```python
from build123d import *

# Parameters (mm, degrees)
SKETCH1_R           = 6.4
BOSS_EXTRUDE1_DEPTH = 77.83
SKETCH2_OUTSIDE_W   = 30.782
SKETCH2_OUTSIDE_H   = 30.782
SKETCH2_OUTSIDE_R   = 3.9
CUT_EXTRUDE1_DEPTH  = 70
CUT_EXTRUDE2_DEPTH  = 5.64
FILLET1_R           = 0.5


with BuildPart() as part:
    # Sketch1 → Boss-Extrude1 (new body)
    with BuildSketch(Plane(origin=(0, 0, 0), x_dir=(1, 0, 0), z_dir=(0, 1, 0))):
        Circle(SKETCH1_R)
    extrude(amount=BOSS_EXTRUDE1_DEPTH)

    # Sketch2 outside → Cut-Extrude1 (cut)
    with BuildSketch(Plane(origin=(0, 77.83, 0), x_dir=(1, 0, 0), z_dir=(0, 1, 0))):
        Rectangle(SKETCH2_OUTSIDE_W, SKETCH2_OUTSIDE_H)
        Circle(SKETCH2_OUTSIDE_R, mode=Mode.SUBTRACT)
    extrude(amount=-CUT_EXTRUDE1_DEPTH, mode=Mode.SUBTRACT)

    # Sketch8 → Cut-Extrude2 (cut)
    with BuildSketch(Plane.XZ):
        Polygon((3.464101615, 0), (1.732050808, 3), (-1.732050808, 3), (-3.464101615, 0), (-1.732050808, -3), (1.732050808, -3), align=None)
    extrude(amount=-CUT_EXTRUDE2_DEPTH, mode=Mode.SUBTRACT)

    # Fillet1
    fillet1_edges = [part.edges().sort_by_distance(p)[0] for p in [
        (-3.9, 77.83, 0),
    ]]
    fillet(fillet1_edges, radius=FILLET1_R)


solid = part.part
```
Geometry check sheet. Reference: the model listing, model coordinates, mm. A direction names the side the tool comes from. Coordinates: 2 decimals unless noted, no trailing zeros. Order: outer loops, then holes, each group sorted by start corner. A loop starts at its lowest first (then second) coordinate and runs counter-clockwise, first axis right, second up. Notation, with made-up numbers: (37.5, 9) - (52.5, 9) arc R26 cw to (52.5, 27) - close; hole circle Ø5 at (17, 29). An arc over 180 degrees is marked (long way). Use one line per item in the form item = value.
1. Access from +Z, -Z, +X, -X, +Y, -Y to the whole of each face (thin tool, end or side, straight path). Record for faces 1 (the face through (-2.87, 43.07, -2.64)), 2 (the face through (-2.6, 2.8, 1.5)), 3 (the face through (0, 77.83, 0)).
Here are the results:
face_1 = +Y
face_2 = -Y
face_3 = +Z, -Z, +X, -X, +Y
2. Draft check along Z on faces 4 (the face through (0, 3, 3)), 5 (the face through (-3, 7.83, 3)), 6 (the face through (-5.08, 3.86, 3.89)). Enter one of: pulls with the +Z half, pulls with the -Z half, needs draft (parallel to the pull), parting line crosses it, or undercut.
Here are the results:
face_4 = undercut
face_5 = needs draft
face_6 = parting line crosses it
3. Section check C-C (z = 5.25). Record the boundary of the cut face in (x, y).
Here are the results:
outline = (-3.66, 0) - (3.66, 0) - (3.66, 7.83) - (-3.66, 7.83) - close
4. Gauge pin test, flat ends, axial feed: pin 1 (2 mm diameter, centred on x = 3, y = 65, fed in from -Z); pin 2 (1 mm diameter, centred on y = 66.5, z = -1.5, fed in from -X); pin 3 (1.5 mm diameter, centred on y = 60.5, z = 0, fed in from -X). Record the tip position at first contact, or that the pin passes through.
Here are the results:
pin_1 = -3.35
pin_2 = -3.77
pin_3 = -3.9
5. Scan lines: line 1 (Y direction, x = -0.25, z = 1); line 2 (X direction, y = 42, z = -3.5); line 3 (Y direction, x = -5, z = 1). Record each from-to range of solid material in increasing order.
Here are the results:
line_1 = 5.64 to 77.83
line_2 = -1.72 to 1.72
line_3 = 0 to 7.83
6. Section check B-B (y = 40). Record the boundary of the cut face in (x, z), then the cut area to 3 significant figures.
Here are the results:
outline = circle Ø7.8 at (0, 0)
area = 47.8 mm²
7. Section check A-A (x = 0). Record the boundary of the cut face in (y, z).
Here are the results:
outline = (0, -6.4) - (7.83, -6.4) - (7.83, -3.9) - (77.33, -3.9) arc R0.5 ccw to (77.83, -3.4) - (77.83, 3.4) arc R0.5 ccw to (77.33, 3.9) - (7.83, 3.9) - (7.83, 6.4) - (0, 6.4) - (0, 3) - (5.64, 3) - (5.64, -3) - (0, -3) - close
